Work out the finished part from the listing and answer in its coordinate system (mm). Face numbers are marked on the shaded views. A direction names the side the tool comes from. Coordinates: 2 decimals unless noted, no trailing zeros. Order: outer loops, then holes, each group sorted by start corner. A loop starts at its lowest first (then second) coordinate and runs counter-clockwise, first axis right, second up.
1. The part is cut by section A-A, the plane x = 0. Give the vertices of the cut face in (y, z), then the cut area to 3 significant figures.
2. Find the intervals of material crossed by probe 1 along X at (y, z) = (0, 104); probe 2 along Z at (x, y) = (-1.5, -4), in increasing order.
3. The part is cut by section C-C, the plane z = 129. Give the vertices of the cut face in (x, y).
4. Flat-ended cylindrical pins translate along their axes: pin 1 Ø1 at (x, z) = (-3, 62) entering from +Y; pin 2 Ø3 at (x, z) = (1.5, 81) entering from +Y; pin 3 Ø4 at (y, z) = (0, 104) entering from -X. Find the tip coordinate at first contact, or state that the pin passes through.
5. A tool of negligible diameter and unlimited length cuts with its end or side. For the marked faces 1 and 2, from which of +Z, -Z, +X, -X, +Y, -Y can it reach the whole face along a straight path? Write none if from no direction.
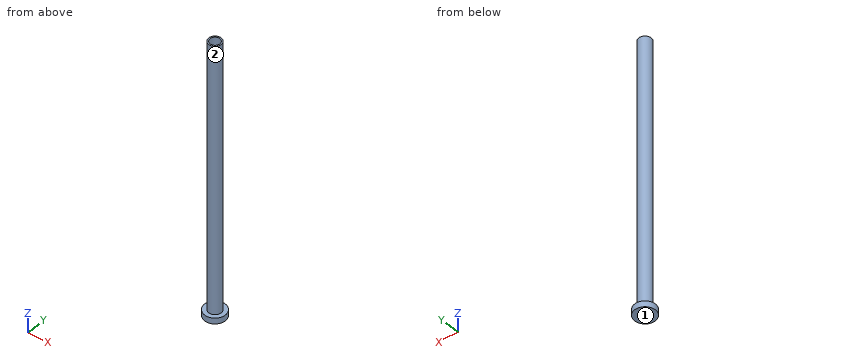
```python
from build123d import *

# Parameters (mm, degrees)
F0_R     = 5.308755
F0_R_2   = 3.2
F0_R_3   = 2.5
F1_DEPTH = 3
F2_DEPTH = 5
F3_DEPTH = 140


with BuildPart() as f1:
    # F0 (on Top) → F1 (new body)
    with BuildSketch(Plane.XY):
        Circle(F0_R)
        Circle(F0_R_2, mode=Mode.SUBTRACT)
        Circle(F0_R_2)
        Circle(F0_R_3, mode=Mode.SUBTRACT)
        Circle(F0_R_3)
    extrude(amount=F1_DEPTH)

    # F0 (on Top) → F2 (join)
    with BuildSketch(Plane.XY):
        Circle(F0_R_2)
        Circle(F0_R_3, mode=Mode.SUBTRACT)
        Circle(F0_R_3)
    extrude(amount=F2_DEPTH)

    # F0 (on Top) → F3 (join)
    with BuildSketch(Plane.XY):
        Circle(F0_R_2)
        Circle(F0_R_3, mode=Mode.SUBTRACT)
    extrude(amount=F3_DEPTH)


solid = f1.part
```
Geometry says:
1. outline: (-5.31, 0) - (5.31, 0) - (5.31, 3) - (3.2, 3) - (3.2, 140) - (2.5, 140) - (2.5, 5) - (-2.5, 5) - (-2.5, 140) - (-3.2, 140) - (-3.2, 3) - (-5.31, 3) - close
1. area: 234 mm2
2. probe 1: x = -3.2 to -2.5, 2.5 to 3.2
2. probe 2: z = 0 to 3
3. outline: circle Ø6.4 at (0, 0); hole circle Ø5 at (0, 0)
4. pin 1: stops at y = 2
4. pin 2: stops at y = 3.2
4. pin 3: stops at x = -3.2
5. face 1: -Z, +X, -X, +Y, -Y
5. face 2: +Z
